Check sheet for the modelled part. Datum: model origin and axes. Units: mm. A direction names the side the tool comes from. Round coordinates to 2 decimals unless told otherwise and drop trailing zeros. Loops run counter-clockwise (first coordinate to the right, second up) from the corner with the lowest first, then second, coordinate; pieces in that order, holes last. Notation, with made-up numbers: (70.5, -20.75) - (106.5, -20.75) arc R15 cw to (106.5, -8.75) - close; hole circle Ø7 at (63.25, 21.5). An arc over 180 degrees is marked (long way). Answer in a Markdown table with one row per item. Add a question column.
(1) Thickness scan on line 1 along Z through (x, y) = (3.75, 19.05); line 2 along X through (y, z) = (109, -15); line 3 along Y through (x, z) = (3.75, -3). Record the ranges inside material, lowest first.
(2) Cross-section at C-C on x = 1.5. Enter the section's corners in (y, z), then the cut area to 3 significant figures.
(3) Cross-section at D-D on y = 93. Enter the section's corners in (x, z).
(4) Cross-section at B-B on y = 19.05. Enter the section's corners in (x, z), then the cut area to 3 significant figures.
(5) Gauge pin test, flat ends, axial feed: pin 1 (6 mm diameter, centred on y = 48.5, z = 21, fed in from -X); pin 2 (1.5 mm diameter, centred on x = 5.5, z = -15.5, fed in from +Y). Record the tip position at first contact, or that the pin passes through.
(6) Mould release check, pull along Z, two halves, no side actions. Record for faces 3 (the cylindrical face through (4.445, 15.384, -26.92)), 4 (the flat face through (7, 55, -38.1)), 5 (the flat face through (6.35, 90, 1)): +Z half, -Z half, draft (parallel to the pull), parting line (faces both ways), or undercut.
(7) Cross-section at A-A on z = -25.4. Enter the section's corners in (x, y).
(8) Access from +Z, -Z, +X, -X, +Y, -Y to the whole of each face (thin tool, end or side, straight path). Record for faces 1 (the flat face through (9.017, 69, 1)), 2 (the flat face through (3, 38.1, 1)).
from build123d import *

# Parameters (mm, degrees)
F1_DEPTH = 38.1
F3_D     = 7.9375


# Not quite as in the source:
# - a length typed as a fraction of an inch, garbled in the dataset ("3 / 203.2 mm" for 3/8 in), is restored


with BuildPart() as f1:
    # F0 (on Top) → F1 (new body, symmetric)
    with BuildSketch(Plane.XY):
        Polygon((0, 38.1), (0, 0), (9.017, 0), (9.017, 139.7), (6.35, 139.7), (6.35, 38.1), align=None)
    extrude(amount=F1_DEPTH, both=True)

    # F3 (through all)
    with Locations(Plane.YZ.offset(9.017)):
        with Locations((19.05, 25.4), (19.05, -25.4)):
            Hole(F3_D / 2)


solid = f1.part
Answers:
| question | item | result |
|---|---|---|
| 1 | line 1 | z = -38.1 to -29.37, -21.43 to 21.43, 29.37 to 38.1 |
| 1 | line 2 | x = 6.35 to 9.02 |
| 1 | line 3 | y = 0 to 38.1 |
| 2 | outline | (0, -38.1) - (38.1, -38.1) - (38.1, 38.1) - (0, 38.1) - close; hole circle Ø7.94 at (19.05, -25.4); hole circle Ø7.94 at (19.05, 25.4) |
| 2 | area | 2,800 mm^2 |
| 3 | outline | (6.35, -38.1) - (9.02, -38.1) - (9.02, 38.1) - (6.35, 38.1) - close |
| 4 | outline | (0, -38.1) - (9.02, -38.1) - (9.02, -29.37) - (0, -29.37) - close; (0, -21.43) - (9.02, -21.43) - (9.02, 21.43) - (0, 21.43) - close; (0, 29.37) - (9.02, 29.37) - (9.02, 38.1) - (0, 38.1) - close |
| 4 | area | 544 mm^2 |
| 5 | pin 1 | stops at x = 6.35 |
| 5 | pin 2 | stops at y = 38.1 |
| 6 | face 3 | undercut |
| 6 | face 4 | -Z half |
| 6 | face 5 | draft |
| 7 | outline | (0, 0) - (9.02, 0) - (9.02, 15.08) - (0, 15.08) - close; (0, 23.02) - (9.02, 23.02) - (9.02, 139.7) - (6.35, 139.7) - (6.35, 38.1) - (0, 38.1) - close |
| 8 | face 1 | +Z, -Z, +X, +Y, -Y |
| 8 | face 2 | +Z, -Z, -X, +Y |
